For this review, take the finished solid that the model builds, in its own axes (mm). Round coordinates to 2 decimals unless told otherwise and drop trailing zeros. Write each loop counter-clockwise with the first axis right and the second up, starting at its lowest first coordinate (ties: lowest second). Pieces come first, ordered by that corner, then holes. Notation, with made-up numbers: M 53,30.25 L 95,30.25 A8 ccw 95,42.25 Z; hole C 6.5,12.5 d10. An arc over 180 degrees is marked long. Answer in a Markdown table with one row per item.
```python
from build123d import *

# Parameters (mm, degrees)
ESQUISSE1_R        = 5
BOSS_EXTRU_1_DEPTH = 3


with BuildPart() as part:
    # Esquisse1 → Boss.-Extru.1 (new body)
    # profile 1 of 3: a face of its own
    with BuildSketch(Plane.XY):
        Polygon((0, 120), (0, 100), (55, 100), (55, 160), (35, 160), align=None)
        with Locations((10, 110)):
            Circle(ESQUISSE1_R, mode=Mode.SUBTRACT)
        with Locations((45, 110)):
            Circle(ESQUISSE1_R, mode=Mode.SUBTRACT)
        with Locations((45, 150)):
            Circle(ESQUISSE1_R, mode=Mode.SUBTRACT)
    # profile 2 of 3: a face of its own
    with BuildSketch(Plane.XY):
        Polygon((55, 100), (0, 100), (0, 0), (90, 0), (90, 5), (200, 5), (200, 80), (200, 100), (145, 100), align=None)
    # profile 3 of 3: a face of its own
    with BuildSketch(Plane.XY):
        Polygon((145, 160), (145, 100), (200, 100), (200, 120), (165, 160), align=None)
        with Locations((155, 110)):
            Circle(ESQUISSE1_R, mode=Mode.SUBTRACT)
        with Locations((190, 110)):
            Circle(ESQUISSE1_R, mode=Mode.SUBTRACT)
        with Locations((155, 150)):
            Circle(ESQUISSE1_R, mode=Mode.SUBTRACT)
    boss_extru_1 = extrude(amount=BOSS_EXTRU_1_DEPTH)

    # Symétrie1: Boss.-Extru.1 across plane
    add(boss_extru_1.mirror(Plane(origin=(0, 0, 3), x_dir=(0, 0, 1), z_dir=(0, 1, 0))))


solid = part.part
```
Q1. For probe 1 along Y at (x, z) = (45, 1.8); probe 2 along X at (y, z) = (-110, 1.2); probe 3 along Y at (x, z) = (111.5, 1.35), list the stretches that pass through material, from the lowest coordinate up.
Found:
| item | result |
|---|---|
| probe 1 | -160 to -155, -145 to -115, -105 to 105, 115 to 145, 155 to 160 |
| probe 2 | 0 to 5, 15 to 40, 50 to 55, 145 to 150, 160 to 185, 195 to 200 |
| probe 3 | -100 to -5, 5 to 100 |
Q2. Mouldability with a two-part tool opening along X and no side actions: class faces 1 (the face through (76, -2, 0)), 2 (the face through (150, -110, 1)), 3 (the face through (17.745, 140.28, 1.479)) as +X half, -X half, draft (parallel to the pull), parting line (faces both ways), or undercut.
Found:
| item | result |
|---|---|
| face 1 | draft |
| face 2 | undercut |
| face 3 | -X half |
Q3. Take a section at A-A (x = 45). State the section outline as (y, z) points, then the cut area to 3 significant figures.
Found:
| item | result |
|---|---|
| outline | M -160,0 L -155,0 L -155,3 L -160,3 Z; M -145,0 L -115,0 L -115,3 L -145,3 Z; M -105,0 L 105,0 L 105,3 L -105,3 Z; M 115,0 L 145,0 L 145,3 L 115,3 Z; M 155,0 L 160,0 L 160,3 L 155,3 Z |
| area | 840 mm² |
Q4. Take a section at B-B (z = 0.75). State how many separate pieces and enclosed holes the cut face has, then the cut area to 3 significant figures.
Found:
| item | result |
|---|---|
| separate pieces | 1 |
| enclosed holes | 12 |
| area | 48,400 mm² |
Q5. Insertion check: P1, Ø8, axis at x = 10, y = -110, coming from the -Z side; P2, Ø1.5, axis at x = 24, z = 1, coming from the +Y side; P3, Ø0.9, axis at y = 1, z = 1.5, coming from the +X side; P4, Ø0.9, axis at x = 124.5, z = 2, coming from the +Y side. Each pin has a flat end and moves straight along its axis. Give the tip position at first contact, or say it passes through.
Found:
| item | result |
|---|---|
| P1 | through |
| P2 | y = 148.29 |
| P3 | x = 90 |
| P4 | y = 100 |
Q6. Take a section at C-C (y = 110). State the section outline as (x, z) points.
Found:
| item | result |
|---|---|
| outline | M 0,0 L 5,0 L 5,3 L 0,3 Z; M 15,0 L 40,0 L 40,3 L 15,3 Z; M 50,0 L 55,0 L 55,3 L 50,3 Z; M 145,0 L 150,0 L 150,3 L 145,3 Z; M 160,0 L 185,0 L 185,3 L 160,3 Z; M 195,0 L 200,0 L 200,3 L 195,3 Z |
Q7. Take a section at D-D (x = 155). State the section outline as (y, z) points, then the cut area to 3 significant figures.
Found:
| item | result |
|---|---|
| outline | M -160,0 L -155,0 L -155,3 L -160,3 Z; M -145,0 L -115,0 L -115,3 L -145,3 Z; M -105,0 L -5,0 L -5,3 L -105,3 Z; M 5,0 L 105,0 L 105,3 L 5,3 Z; M 115,0 L 145,0 L 145,3 L 115,3 Z; M 155,0 L 160,0 L 160,3 L 155,3 Z |
| area | 810 mm² |
